CAD build for the part. Positions are in the model's coordinates, mm. A direction names the side the tool comes from. Round coordinates to 2 decimals unless told otherwise and drop trailing zeros. Loops run counter-clockwise (first coordinate to the right, second up) from the corner with the lowest first, then second, coordinate; pieces in that order, holes last. Notation, with made-up numbers: (19, 11.5) - (34, 11.5) arc R20 ccw to (34, 43.5) - close; hole circle Ø6 at (85.25, 25.25). An arc over 180 degrees is marked (long way). Use one line per item in the form item = value.
from build123d import *

# Parameters (mm, degrees)
ESQUISSE1_R        = 19.95
ESQUISSE1_R_2      = 5
ESQUISSE1_R_3      = 2.5
BOSS_EXTRU_1_DEPTH = 4
ESQUISSE2_R        = 25
ESQUISSE2_R_2      = 2.5
ESQUISSE2_R_3      = 5
BOSS_EXTRU_2_DEPTH = 6


with BuildPart() as part:
    # Esquisse1 → Boss.-Extru.1 (new body)
    with BuildSketch(Plane(origin=(0, 0, 0), x_dir=(1, 0, 0), z_dir=(0, 1, 0))):
        Circle(ESQUISSE1_R)
        Circle(ESQUISSE1_R_2, mode=Mode.SUBTRACT)
        with Locations((0, 12.5)):
            Circle(ESQUISSE1_R_3, mode=Mode.SUBTRACT)
        with Locations((10.825317547, 6.25)):
            Circle(ESQUISSE1_R_3, mode=Mode.SUBTRACT)
        with Locations((10.825317547, -6.25)):
            Circle(ESQUISSE1_R_3, mode=Mode.SUBTRACT)
        with Locations((0, -12.5)):
            Circle(ESQUISSE1_R_3, mode=Mode.SUBTRACT)
        with Locations((-10.825317547, -6.25)):
            Circle(ESQUISSE1_R_3, mode=Mode.SUBTRACT)
        with Locations((-10.825317547, 6.25)):
            Circle(ESQUISSE1_R_3, mode=Mode.SUBTRACT)
    extrude(amount=BOSS_EXTRU_1_DEPTH)

    # Esquisse2 → Boss.-Extru.2 (add)
    with BuildSketch(Plane(origin=(0, 4, 0), x_dir=(1, 0, 0), z_dir=(0, 1, 0))):
        Circle(ESQUISSE2_R)
        with Locations((0, 12.5)):
            Circle(ESQUISSE2_R_2, mode=Mode.SUBTRACT)
        with Locations((10.825317547, 6.25)):
            Circle(ESQUISSE2_R_2, mode=Mode.SUBTRACT)
        with Locations((10.825317547, -6.25)):
            Circle(ESQUISSE2_R_2, mode=Mode.SUBTRACT)
        Circle(ESQUISSE2_R_3, mode=Mode.SUBTRACT)
        with Locations((0, -12.5)):
            Circle(ESQUISSE2_R_2, mode=Mode.SUBTRACT)
        with Locations((-10.825317547, -6.25)):
            Circle(ESQUISSE2_R_2, mode=Mode.SUBTRACT)
        with Locations((-10.825317547, 6.25)):
            Circle(ESQUISSE2_R_2, mode=Mode.SUBTRACT)
    extrude(amount=BOSS_EXTRU_2_DEPTH)


solid = part.part
1) Slice it at D-D (z = 6.25). Write the cut outline in (x, y).
Report:
outline = (-24.21, 4) - (-18.95, 4) - (-18.95, 0) - (-13.33, 0) - (-13.33, 10) - (-24.21, 10) - close; (-8.33, 0) - (8.33, 0) - (8.33, 10) - (-8.33, 10) - close; (13.33, 0) - (18.95, 0) - (18.95, 4) - (24.21, 4) - (24.21, 10) - (13.33, 10) - close
2) Slice it at A-A (z = 0). Write the cut outline in (x, y).
Report:
outline = (-25, 4) - (-19.95, 4) - (-19.95, 0) - (-5, 0) - (-5, 10) - (-25, 10) - close; (5, 0) - (19.95, 0) - (19.95, 4) - (25, 4) - (25, 10) - (5, 10) - close
3) Drill centre lines: probe 1 along Z at (x, y) = (0, 2.75); probe 2 along X at (y, z) = (3.25, -6.25); probe 3 along Z at (x, y) = (0, 7). Where is each one in solid material? Low to high.
Report:
probe_1 = -19.95 to -15, -10 to -5, 5 to 10, 15 to 19.95
probe_2 = -18.95 to -13.33, -8.33 to 8.33, 13.33 to 18.95
probe_3 = -25 to -15, -10 to -5, 5 to 10, 15 to 25
4) Flat gauge pins, fed straight in: pin 1 (2 mm diameter, centred on y = 3.5, z = -6.5, fed in from +X); pin 2 (5 mm diameter, centred on x = -18.5, y = 8.5, fed in from +Z); pin 3 (1.5 mm diameter, centred on y = 5, z = 8, fed in from +X). Where does each tip first touch, or does it go through?
Report:
pin_1 = 24.36
pin_2 = 19.21
pin_3 = 23.93
5) Slice it at B-B (y = 3.25). Write the cut outline in (x, z).
Report:
outline = circle Ø39.9 at (0, 0); hole circle Ø5 at (-10.83, -6.25); hole circle Ø5 at (-10.83, 6.25); hole circle Ø10 at (0, 0); hole circle Ø5 at (0, -12.5); hole circle Ø5 at (0, 12.5); hole circle Ø5 at (10.83, -6.25); hole circle Ø5 at (10.83, 6.25)
6) Two-plate mould, pull along Z, no slides. Class faces 1 (the flat face through (4, 0, 4)), 2 (the cylindrical face through (-8.44, 4.93, -7)), 3 (the cylindrical face through (23.846, 6.958, -7.509)): +Z half, -Z half, draft (parallel to the pull), parting line (faces both ways), or undercut.
Report:
face_1 = draft
face_2 = undercut
face_3 = parting line
7) Slice it at C-C (x = 0). Write the cut outline in (y, z).
Report:
outline = (0, -19.95) - (4, -19.95) - (4, -25) - (10, -25) - (10, -15) - (0, -15) - close; (0, -10) - (10, -10) - (10, -5) - (0, -5) - close; (0, 5) - (10, 5) - (10, 10) - (0, 10) - close; (0, 15) - (10, 15) - (10, 25) - (4, 25) - (4, 19.95) - (0, 19.95) - close
8) Tool access for faces 4 (the cylindrical face through (13.21, 4.93, 5.5)), 5 (the flat face through (-17, 4, 11)): list every direction of +Z, -Z, +X, -X, +Y, -Y with a clear straight run to the whole face (end or side of a thin tool).
Report:
face_4 = +Y, -Y
face_5 = -Y
